Source: CAD feature listing. Evaluate the final solid. Frame: model axes, mm. Face numbers are marked on the shaded views. A direction names the side the tool comes from. Give positions to 0.01 mm unless a question says otherwise; leave off trailing zeros. Write each loop counter-clockwise with the first axis right and the second up, starting at its lowest first coordinate (ties: lowest second). Pieces come first, ordered by that corner, then holes.
```python
from build123d import *

# Parameters (mm, degrees)
F0_W      = 76.2
F0_H      = 76.2
F1_DEPTH  = 63.5
F2_W      = 68.58
F2_H      = 68.58
F3_DEPTH  = 54.356
F4_W      = 76.2
F4_H      = 12.7
F5_DEPTH  = 12.7
F7_DEPTH  = 81.788
F8_R      = 5.08
F9_W      = 66.04
F9_H      = 20.32
F10_DEPTH = 25.4
F12_DEPTH = 25.4
F13_W     = 8.3356503789
F13_H     = 20.32
F14_DEPTH = 17.78
F15_W     = 2.54
F15_H     = 20.32
F16_DEPTH = 27.178
F17_W     = 2.54
F17_H     = 20.32
F18_DEPTH = 29.972
F20_DEPTH = 4.826


with BuildPart() as f1:
    # F0 (on Front) → F1 (new body)
    with BuildSketch(Plane.XZ):
        with Locations((-1.4287489414, -3.7570823967)):
            Rectangle(F0_W, F0_H)
    extrude(amount=F1_DEPTH)

    # F2 (on face) → F3 (cut)
    with BuildSketch(Plane.XZ.offset(63.5)):
        with Locations((-1.5081233764, -2.9368781066)):
            Rectangle(F2_W, F2_H)
    extrude(amount=-F3_DEPTH, mode=Mode.SUBTRACT)

    # F4 (on face) → F5 (join)
    with BuildSketch(Plane(origin=(0, 0, -41.8570823967), x_dir=(1, 0, 0), z_dir=(0, 0, -1))):
        with Locations((-1.4287489414, 6.35)):
            Rectangle(F4_W, F4_H)
    extrude(amount=F5_DEPTH)

    # F6 (on face) → F7 (cut)
    with BuildSketch(Plane(origin=(-39.5287489414, 0, 0), x_dir=(0, -1, 0), z_dir=(-1, 0, 0))):
        Polygon((12.7, -48.2070823967), (0, -54.5570823967), (12.7, -54.5570823967), align=None)
    extrude(amount=-F7_DEPTH, mode=Mode.SUBTRACT)

    # F8
    f8_edges = [f1.edges().sort_by_distance(p)[0] for p in [
        (-39.528749, -38.1, -41.857082),
        (36.671251, -38.1, -41.857082),
        (-1.428749, -12.7, -48.207082),
        (-39.528749, -12.7, -45.032082),
        (36.671251, -12.7, -45.032082),
        (36.671251, -31.75, 34.342918),
        (-39.528749, -31.75, 34.342918),
    ]]
    fillet(f8_edges, radius=F8_R)

    # F9 (on face) → F10 (cut)
    with BuildSketch(Plane(origin=(0, 0, 0), x_dir=(-1, 0, 0), z_dir=(0, 1, 0))):
        with Locations((1.4287489414, 19.1029176033)):
            Rectangle(F9_W, F9_H)
    extrude(amount=-F10_DEPTH, mode=Mode.SUBTRACT)

    # F11 (on face) → F12 (join)
    with BuildSketch(Plane(origin=(0, 0, 29.2629176033), x_dir=(1, 0, 0), z_dir=(0, 0, -1))):
        Polygon((4.1656, 9.144), (-4.1700503789, 9.144), (-4.1700503789, 0), (0, 0), (4.1656, 0), align=None)
    extrude(amount=F12_DEPTH)

    # F13 (on face) → F14 (join)
    with BuildSketch(Plane(origin=(0, 0, 0), x_dir=(-1, 0, 0), z_dir=(0, 1, 0))):
        with Locations((0.0022251894, 19.1029176033)):
            Rectangle(F13_W, F13_H)
    extrude(amount=F14_DEPTH)

    # F15 (on face) → F16 (join)
    with BuildSketch(Plane.YZ.offset(4.1656)):
        with Locations((16.51, 19.1029176033)):
            Rectangle(F15_W, F15_H)
    extrude(amount=F16_DEPTH)

    # F17 (on face) → F18 (join)
    with BuildSketch(Plane(origin=(-4.1700503789, 0, 0), x_dir=(0, -1, 0), z_dir=(-1, 0, 0))):
        with Locations((-16.51, 19.1029176033)):
            Rectangle(F17_W, F17_H)
    extrude(amount=F18_DEPTH)

    # F19 (on face) → F20 (join)
    with BuildSketch(Plane(origin=(0, 0, 0), x_dir=(-1, 0, 0), z_dir=(0, 1, 0))):
        with BuildLine():
            ThreePointArc((39.5287489414, 29.2629176033), (38.0408513898, 32.8550200517), (34.4487489414, 34.3429176033))
            Line((34.4487489414, 34.3429176033), (-31.5912510586, 34.3429176033))
            ThreePointArc((-31.5912510586, 34.3429176033), (-35.183353507, 32.8550200517), (-36.6712510586, 29.2629176033))
            Line((-36.6712510586, 29.2629176033), (-36.6712510586, -54.5570823967))
            Line((-36.6712510586, -54.5570823967), (39.5287489414, -54.5570823967))
            Line((39.5287489414, -54.5570823967), (39.5287489414, 29.2629176033))
        make_face()
        Polygon((34.4487489414, 29.2629176033), (34.4487489414, 8.9429176033), (4.1700503789, 8.9429176033), (-4.1656, 8.9429176033), (-31.5912510586, 8.9429176033), (-31.5912510586, 29.2629176033), (-4.1656, 29.2629176033), (4.1700503789, 29.2629176033), align=None, mode=Mode.SUBTRACT)
    extrude(amount=F20_DEPTH)


solid = f1.part
```
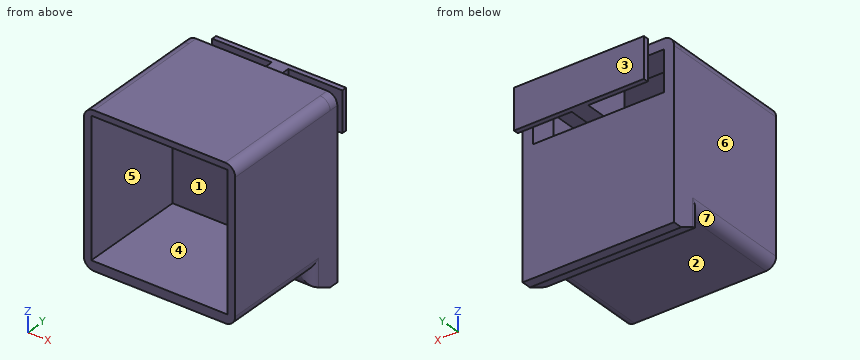
1. Section query D-D (x = 1). Return loops of the section in (y, z), plus the area to 3 significant figures.
2. Section query C-C (y = -48). Return loops of the section in (x, z).
3. Access query for the marked faces 5, 6 and 7. Directions: +Z, -Z, +X, -X, +Y, -Y. A direction counts if a zero-diameter tool reaches every point of the face in a straight line with its end or side. Return the directions, or none.
4. Section query B-B (x = -11). Return loops of the section in (y, z).
5. Section query A-A (z = 12). Return loops of the section in (x, y), plus the area to 3 significant figures.
6. Line query: probe 1 along X at (y, z) = (-3.5, 16); probe 2 along Z at (x, y) = (-30.5, -24.5); probe 3 along X at (y, z) = (-22.5, -24.5). Output: solid intervals per line, ascending.
7. Pull-direction query (Z, two-part tool) for the marked faces 1, 2, 3 and 4; classes: pulls with the +Z half, pulls with the -Z half, needs draft (parallel to the pull), parting line crosses it, or undercut.
8. Pin query (flat end, axial travel): P1, Ø12, axis at x = -6.5, y = -14.5, coming from the -Z side; P2, Ø7, axis at x = -26, y = -5.5, coming from the -Z side; P3, Ø6, axis at x = -7.5, y = -45, coming from the -Z side. Return the tip coordinate at first contact, or that it passes through.
The answers:
1. outline: (-63.5, -41.86) - (-12.7, -41.86) - (-12.7, -45.07) arc R5.08 ccw to (-9.89, -49.61) - (0, -54.56) - (4.83, -54.56) - (4.83, 8.94) - (17.78, 8.94) - (17.78, 29.26) - (4.83, 29.26) - (4.83, 34.34) - (-63.5, 34.34) - (-63.5, 31.35) - (-9.14, 31.35) - (-9.14, -37.23) - (-63.5, -37.23) - close
1. area: 1,920 mm2
2. outline: (-39.53, -36.78) arc R5.08 ccw to (-34.45, -41.86) - (31.59, -41.86) arc R5.08 ccw to (36.67, -36.78) - (36.67, 29.26) arc R5.08 ccw to (31.59, 34.34) - (-34.45, 34.34) arc R5.08 ccw to (-39.53, 29.26) - close; hole (-35.8, -37.23) - (32.78, -37.23) - (32.78, 31.35) - (-35.8, 31.35) - close
3. face 5: -Y
3. face 6: +Z, -Z, -X, +Y, -Y
3. face 7: -Z, -X, -Y
4. outline: (-63.5, -41.86) - (-12.7, -41.86) - (-12.7, -45.07) arc R5.08 ccw to (-9.89, -49.61) - (0, -54.56) - (4.83, -54.56) - (4.83, 8.94) - (-9.14, 8.94) - (-9.14, -37.23) - (-63.5, -37.23) - close; (-63.5, 31.35) - (-9.14, 31.35) - (-9.14, 29.26) - (4.83, 29.26) - (4.83, 34.34) - (-63.5, 34.34) - close; (15.24, 8.94) - (17.78, 8.94) - (17.78, 29.26) - (15.24, 29.26) - close
5. outline: (-39.53, -63.5) - (-35.8, -63.5) - (-35.8, -9.14) - (-34.45, -9.14) - (-34.45, 4.83) - (-39.53, 4.83) - close; (-34.14, 15.24) - (-4.17, 15.24) - (-4.17, -9.14) - (4.17, -9.14) - (4.17, 15.24) - (31.34, 15.24) - (31.34, 17.78) - (-34.14, 17.78) - close; (31.59, -9.14) - (32.78, -9.14) - (32.78, -63.5) - (36.67, -63.5) - (36.67, 4.83) - (31.59, 4.83) - close
5. area: 926 mm2
6. probe 1: x = -39.53 to -34.45, -4.17 to 4.17, 31.59 to 36.67
6. probe 2: z = -41.86 to -37.23, 31.35 to 34.34
6. probe 3: x = -39.53 to -35.8, 32.78 to 36.67
7. face 1: undercut
7. face 2: pulls with the -Z half
7. face 3: needs draft
7. face 4: undercut
8. P1: stops at z = -50.31
8. P2: stops at z = -53.56
8. P3: stops at z = -41.86
